Input: part model. Units: mm. Frame: model coordinates. A direction names the side the tool comes from. Give positions to 0.01 mm unless a question says otherwise; leave off trailing zeros. Loops run counter-clockwise (first coordinate to the right, second up) from the corner with the lowest first, then second, coordinate; pieces in that order, holes last. Notation, with made-up numbers: (52, -28) - (95, -28) arc R22 cw to (95, -17) - close; hole circle Ø10 at (64, 15.5). An arc over 180 degrees is marked (long way). Answer as a JSON object with one key per item and string values. Group by question number.
(1) Mould query, pull axis X, two halves, no side actions, for faces 1 (the flat face through (-6, 2, 3)), 2 (the flat face through (6, 2, 3)), 3 (the flat face through (5, 2, 5)), 4 (the flat face through (-2, 2, 4)). Classes: +X half, -X half, draft (parallel to the pull), parting line (faces both ways), or undercut.
(2) Access query for faces 5 (the flat face through (3, -2, 1)), 6 (the flat face through (-5, 2, 5)), 7 (the cylindrical face through (-4.48, -4.07, 0.45)), 8 (the cylindrical face through (4.52, -4.07, 0.45)). Directions: +Z, -Z, +X, -X, +Y, -Y. A direction counts if a zero-diameter tool reaches every point of the face in a straight line with its end or side. Return the directions, or none.
(3) Section query A-A (x = -4.5). Return loops of the section in (y, z).
(4) Section query C-C (z = 5.5). Return loops of the section in (x, y).
(5) Section query B-B (y = 3.25). Return loops of the section in (x, z).
(6) Material intervals for L1, parallel to X at y = -2, z = 3; L2, parallel to X at y = 2.75, z = 2.75; L3, parallel to Z at x = -2.5, y = -2, sorted ascending.
(7) Pin query (flat end, axial travel): P1, Ø1.1, axis at x = -3, z = 5, coming from the +Y side; P2, Ø1.5, axis at x = -1.5, z = 1, coming from the -Y side; P3, Ø0.9, axis at x = -2, y = -0.5, coming from the -Z side; P4, Ø0.8, axis at y = -1, z = 3, coming from the -X side. Return the tip coordinate at first contact, or that it passes through.
(8) Section query D-D (z = 3.75). Count the separate pieces of the cut face and the enclosed holes in it, plus the area to 3 significant figures.
```python
from build123d import *

# Parameters (mm, degrees)
F0_W          = 12
F0_H          = 9
F1_DEPTH      = 6
F2_W          = 3
F2_H          = 6
F3_DEPTH      = 3.5
F4_W          = 6
F4_H          = 6.5
F5_DEPTH      = 3.5
F6_R          = 1.25
F7_DEPTH      = 3
F8_R          = 1.25
F9_DEPTH      = 3.001
F10_R         = 1.5
F11_W         = 2.5
F11_H         = 6.5
F12_DEPTH     = 2.75
F13_R         = 1.1
F14_T8_ANGLE  = 247.5355258221
F14_T13_ANGLE = 80.8755372564
F14_T18_ANGLE = 260.9918579461
F14_T24_ANGLE = 247.5355258221
F14_T29_ANGLE = 260.9918579461
F14_T35_ANGLE = 80.8755372564


# Not quite as in the source:
# - a fillet or chamfer that OpenCascade refuses, or shapes differently, is made with other operations: its cross-section is extruded or revolved along the edge and cut away or added


with BuildPart() as f1:
    # F0 (on Top) → F1 (new body)
    with BuildSketch(Plane.XY):
        Rectangle(F0_W, F0_H)
    extrude(amount=F1_DEPTH)

    # F2 (on face) → F3 (cut)
    with BuildSketch(Plane.XY.offset(6)):
        with Locations((3.5, 1.5)):
            Rectangle(F2_W, F2_H)
        with Locations((-3.5, 1.5)):
            Rectangle(F2_W, F2_H)
    extrude(amount=-F3_DEPTH, mode=Mode.SUBTRACT)

    # F4 (on face) → F5 (cut)
    with BuildSketch(Plane(origin=(0, 0, 0), x_dir=(1, 0, 0), z_dir=(0, 0, -1))):
        with Locations((0, 1.25)):
            Rectangle(F4_W, F4_H)
    extrude(amount=-F5_DEPTH, mode=Mode.SUBTRACT)

    # F6 (on face) → F7 (cut)
    with BuildSketch(Plane.YZ.offset(6)):
        with Locations((0, 3)):
            Circle(F6_R)
    extrude(amount=-F7_DEPTH, mode=Mode.SUBTRACT)

    # F8 (on face) → F9 (cut, through all)
    with BuildSketch(Plane(origin=(-6, 0, 0), x_dir=(0, -1, 0), z_dir=(-1, 0, 0))):
        with Locations((0, 3)):
            Circle(F8_R)
    extrude(amount=-F9_DEPTH, mode=Mode.SUBTRACT)

    # F10
    f10_edges = [f1.edges().sort_by_distance(p)[0] for p in [
        (2, 1.5, 6),
        (-2, 1.5, 6),
        (0, -4.5, 6),
        (-4.5, -4.5, 0),
        (4.5, -4.5, 0),
        (0, 4.5, 0),
        (-5.5, 4.5, 6),
        (5.5, 4.5, 6),
        (0, 4.5, 6),
    ]]
    fillet(f10_edges, radius=F10_R)

    # F11 (on face) → F12 (join)
    with BuildSketch(Plane(origin=(0, 0, 3.5), x_dir=(1, 0, 0), z_dir=(0, 0, -1))):
        with Locations((0, 1.25)):
            Rectangle(F11_W, F11_H)
    extrude(amount=F12_DEPTH)

    # F13
    f13_edges = [f1.edges().sort_by_distance(p)[0] for p in [
        (-1.25, -1.25, 0.75),
        (1.25, -1.25, 0.75),
    ]]
    fillet(f13_edges, radius=F13_R)

    # F14: fillet of radius 0.5 on 7 edges, made by hand

    # F14_s1 → F14_t2 (revolve, cut)
    with BuildSketch(Plane.XY.offset(3)):
        with BuildLine():
            ThreePointArc((6, 1.75), (5.8535533906, 1.3964466094), (5.5, 1.25))
            Line((5.5, 1.25), (6, 1.25))
            Line((6, 1.25), (6, 1.75))
        make_face()
    revolve(axis=Axis((6, 0, 3), (1, 0, 0)), mode=Mode.SUBTRACT)

    # F14_s3 → F14_t4 (revolve, cut)
    with BuildSketch(Plane.XY.offset(3)):
        with BuildLine():
            ThreePointArc((-6, -1.75), (-5.8535533906, -1.3964466094), (-5.5, -1.25))
            Line((-5.5, -1.25), (-6, -1.25))
            Line((-6, -1.25), (-6, -1.75))
        make_face()
    revolve(axis=Axis((-6, 0, 3), (-1, 0, 0)), mode=Mode.SUBTRACT)


with BuildPart() as f14_tool6:
    # F14_s7 → F14_t8 (revolve)
    with BuildSketch(Plane(origin=(0, -1.3861749524, 2.0731657713), x_dir=(1, 0, 0), z_dir=(0, -0.5558279796, 0.8312973338))):
        with BuildLine():
            ThreePointArc((-3, 3.4174839388), (-3.1464466094, 3.0639305482), (-3.5, 2.9174839388))
            Line((-3.5, 2.9174839388), (-3, 2.9174839388))
            Line((-3, 2.9174839388), (-3, 3.4174839388))
        make_face()
    revolve(axis=Axis((-3, 0, 3), (-1, 0, 0)), revolution_arc=F14_T8_ANGLE)

    split(bisect_by=Plane.XY.offset(3.5), keep=Keep.BOTTOM)


with BuildPart() as f1_1:
    add(f1.part)

    # F14_t5: cut F14_tool6
    add(f14_tool6.part, mode=Mode.SUBTRACT)


with BuildPart() as f14_tool11:
    # F14_s12 → F14_t13 (revolve)
    with BuildSketch(Plane(origin=(0, 0.469718994, 0.0754425014), x_dir=(1, 0, 0), z_dir=(0, -0.9873461903, -0.1585796345))):
        with BuildLine():
            ThreePointArc((5.5, 1.7120385709), (5.1464466094, 1.5655919615), (5, 1.2120385709))
            Line((5, 1.2120385709), (5, 1.7120385709))
            Line((5, 1.7120385709), (5.5, 1.7120385709))
        make_face()
    revolve(axis=Axis((5, 0, 3), (1, 0, 0)), revolution_arc=F14_T13_ANGLE)

    split(bisect_by=Plane.XY.offset(2.5), keep=Keep.TOP)


with BuildPart() as f1_2:
    add(f1_1.part)

    # F14_t10: cut F14_tool11
    add(f14_tool11.part, mode=Mode.SUBTRACT)


with BuildPart() as f14_tool16:
    # F14_s17 → F14_t18 (revolve)
    with BuildSketch(Plane.XY.offset(3)):
        with BuildLine():
            ThreePointArc((5.5, 1.25), (5.1464466094, 1.3964466094), (5, 1.75))
            Line((5, 1.75), (5, 1.25))
            Line((5, 1.25), (5.5, 1.25))
        make_face()
    revolve(axis=Axis((5, 0, 3), (1, 0, 0)), revolution_arc=F14_T18_ANGLE)

    split(bisect_by=Plane.XZ.offset(1.5), keep=Keep.BOTTOM)

    split(bisect_by=Plane.XY.offset(2.5), keep=Keep.TOP)


with BuildPart() as f1_3:
    add(f1_2.part)

    # F14_t15: cut F14_tool16
    add(f14_tool16.part, mode=Mode.SUBTRACT)


with BuildPart() as f14_tool22:
    # F14_s23 → F14_t24 (revolve)
    with BuildSketch(Plane(origin=(0, 1.3861749524, 2.0731657713), x_dir=(1, 0, 0), z_dir=(0, 0.5558279796, 0.8312973338))):
        with BuildLine():
            ThreePointArc((3, -3.4174839388), (3.1464466094, -3.0639305482), (3.5, -2.9174839388))
            Line((3.5, -2.9174839388), (3, -2.9174839388))
            Line((3, -2.9174839388), (3, -3.4174839388))
        make_face()
    revolve(axis=Axis((3, 0, 3), (1, 0, 0)), revolution_arc=F14_T24_ANGLE)

    split(bisect_by=Plane.XY.offset(3.5), keep=Keep.BOTTOM)


with BuildPart() as f1_4:
    add(f1_3.part)

    # F14_t21: cut F14_tool22
    add(f14_tool22.part, mode=Mode.SUBTRACT)


with BuildPart() as f14_tool27:
    # F14_s28 → F14_t29 (revolve)
    with BuildSketch(Plane.XY.offset(3)):
        with BuildLine():
            ThreePointArc((-5.5, -1.25), (-5.1464466094, -1.3964466094), (-5, -1.75))
            Line((-5, -1.75), (-5, -1.25))
            Line((-5, -1.25), (-5.5, -1.25))
        make_face()
    revolve(axis=Axis((-5, 0, 3), (-1, 0, 0)), revolution_arc=F14_T29_ANGLE)

    split(bisect_by=Plane.XZ.offset(1.5), keep=Keep.BOTTOM)

    split(bisect_by=Plane.XY.offset(2.5), keep=Keep.TOP)


with BuildPart() as f1_5:
    add(f1_4.part)

    # F14_t26: cut F14_tool27
    add(f14_tool27.part, mode=Mode.SUBTRACT)


with BuildPart() as f14_tool33:
    # F14_s34 → F14_t35 (revolve)
    with BuildSketch(Plane(origin=(0, -0.469718994, 0.0754425014), x_dir=(1, 0, 0), z_dir=(0, 0.9873461903, -0.1585796345))):
        with BuildLine():
            ThreePointArc((-5.5, -1.7120385709), (-5.1464466094, -1.5655919615), (-5, -1.2120385709))
            Line((-5, -1.2120385709), (-5, -1.7120385709))
            Line((-5, -1.7120385709), (-5.5, -1.7120385709))
        make_face()
    revolve(axis=Axis((-5, 0, 3), (-1, 0, 0)), revolution_arc=F14_T35_ANGLE)

    split(bisect_by=Plane.XZ.offset(1.5), keep=Keep.BOTTOM)

    split(bisect_by=Plane.XY.offset(2.5), keep=Keep.TOP)


with BuildPart() as f1_6:
    add(f1_5.part)

    # F14_t32: cut F14_tool33
    add(f14_tool33.part, mode=Mode.SUBTRACT)


solid = f1_6.part
```
Recorded:
{
 "1": {"face 1": "-X half", "face 2": "+X half", "face 3": "undercut", "face 4": "undercut"},
 "2": {"face 5": "-Z, -Y", "face 6": "+Z, +Y", "face 7": "-Z, -X, -Y", "face 8": "-Z, +X, -Y"},
 "3": {"outline": "(-4.5, 1.5) arc R1.5 ccw to (-3, 0) - (3, 0) arc R1.5 ccw to (4.5, 1.5) - (4.5, 2.5) - (1.15, 2.5) arc R1.25 cw to (-1.15, 2.5) - (-1.5, 2.5) - (-1.5, 6) - (-3, 6) arc R1.5 ccw to (-4.5, 4.5) - close"},
 "4": {"outline": "(-6, -4.12) - (6, -4.12) - (6, 4.12) - (5, 4.12) - (5, -1.5) - (1.62, -1.5) - (1.62, 4.12) - (-1.62, 4.12) - (-1.62, -1.5) - (-5, -1.5) - (-5, 4.12) - (-6, 4.12) - close"},
 "5": {"outline": "(-6, 0.02) - (6, 0.02) - (6, 5.98) - (5, 5.98) - (5, 2.5) - (2, 2.5) - (2, 4.5) arc R1.5 ccw to (0.75, 5.98) - (-0.75, 5.98) arc R1.5 ccw to (-2, 4.5) - (-2, 2.5) - (-5, 2.5) - (-5, 5.98) - (-6, 5.98) - close"},
 "6": {"L1": "x = -6 to -3, -1.25 to 1.25, 3 to 6", "L2": "x = -6 to -5, -2 to 2, 5 to 6", "L3": "z = 3.5 to 6"},
 "7": {"P1": "stops at y = -1.5", "P2": "stops at y = -4.5", "P3": "stops at z = 3.5", "P4": "stops at x = -5.86"},
 "8": {"separate pieces": "3", "enclosed holes": "0", "area": "67.5 mm^2"}
}
